Autodesk Inventor part; units mm, degrees
ref_plane "YZ Plane" through (0, 0, 0) normal (1, 0, 0) x (0, 1, 0)
ref_plane "XZ Plane" through (0, 0, 0) normal (0, 1, 0) x (-1, 0, 0)
ref_plane "XY Plane" through (0, 0, 0) normal (0, 0, 1) x (1, 0, 0)
sketch "Sketch1" plane through (0, 0, 0) normal (0, 0, 1) x (1, 0, 0)
  line L0 (-41.148, 14.2875) -> (41.148, 14.2875)
  line L1 (41.148, 14.2875) -> (41.148, -14.2875)
  line L2 (41.148, -14.2875) -> (-41.148, -14.2875)
  line L3 (-41.148, -14.2875) -> (-41.148, 14.2875)
  point P0 (0, 0)
  dimension "d0" = 82.296
  dimension "d1" = 41.148
  dimension "d2" = 14.2875
  dimension "d3" = 28.575
extrude "Extrusion1" add sketch "Sketch1" along normal mid plane 6.35
sketch "Sketch2" plane through (0, 0, 3.175) normal (0, 0, 1) x (1, 0, 0)
  circle A0 centre (-25.781, 0) radius 11.303
  circle A1 centre (0, 0) radius 11.303
  line L0 (41.148, -14.2875) -> (41.148, 14.2875)
  circle A2 centre (25.781, 0) radius 11.303
  line L1 (-41.148, 14.2875) -> (-41.148, -14.2875)
  line L2 (-41.148, 0) -> (41.148, 0) construction
  line L3 (41.148, 14.2875) -> (-41.148, 14.2875)
  point P0 (0, 0)
  dimension "d6" = 22.606
  dimension "d9" = 22.606
  dimension "d11" = 22.606
  dimension "d14" = 25.781
  dimension "d21" = 82.296
  dimension "d22" = 25.781
  dimension "d50" = 0
  dimension "d150" = 3.175
sketch "Sketch4" plane through (-41.148, -14.2875, -3.175) normal (-1, 0, 0) x (0, 0, 1)
  line L0 (0, 0) -> (0, 28.575)
  line L1 (6.35, 28.575) -> (6.35, 0)
  line L2 (0, 22.6695) -> (6.35, 22.6695)
  line L3 (6.35, 22.6695) -> (6.35, 5.9055)
  line L4 (6.35, 5.9055) -> (0, 5.9055)
  line L5 (0, 5.9055) -> (0, 22.6695)
  point P0 (3.175, 14.2875)
  dimension "d30" = 8.382
  dimension "d31" = 16.764
extrude "Extrusion3" cut sketch "Sketch4" against normal blind 0.635
mirror "Mirror1" about plane through (0, 0, 0) normal (1, 0, 0) of "Extrusion3"
sketch "Sketch5" plane through (0, 0, 3.175) normal (0, 0, 1) x (1, 0, 0)
  circle A0 centre (0, 9.7155) radius 3.175 construction
  line L0 (41.148, 14.2875) -> (-41.148, 14.2875)
  line L1 (-18.3944, 20.454) -> (40.513, 0) construction
  line L2 (40.513, 8.382) -> (40.513, -8.382)
  circle A1 centre (2.6968, 17.4822) radius 3.175 construction
  circle A2 centre (35.941, 1.5875) radius 3.175 construction
  circle A3 centre (-35.941, 26.5465) radius 3.175 construction
  line L3 (-40.513, 8.382) -> (-40.513, -8.382)
  circle A4 centre (36.576, 9.7155) radius 3.175
  circle A5 centre (-36.576, -9.7155) radius 3.175
  line L4 (41.148, 8.382) -> (41.148, 14.2875)
  line L5 (-41.148, -14.2875) -> (41.148, -14.2875)
  line L6 (-41.148, -14.2875) -> (-41.148, -8.382)
  point P0 (0, 0)
  dimension "d34" = 6.35
  dimension "d35" = 4.572
  dimension "d53" = 6.35
  dimension "d54" = 6.35
  dimension "d55" = 4.572
  dimension "d56" = 4.572
  dimension "d57" = 12.7
  dimension "d58" = 6.35
  dimension "d59" = 6.35
  dimension "d60" = 4.572
  dimension "d61" = 4.572
  dimension "d62" = 4.572
  dimension "d63" = 4.572
extrude "Extrusion4" cut sketch "Sketch5" against normal blind 1.27
sketch "Sketch7" plane through (-41.148, -14.2875, 3.175) normal (0, -1, 0) x (1, 0, 0)
  line L0 (27.178, -14.605) -> (55.118, -14.605)
  line L1 (55.118, -14.605) -> (55.118, 8.255)
  line L2 (55.118, 8.255) -> (27.178, 8.255)
  line L3 (27.178, 8.255) -> (27.178, -14.605)
  point P0 (41.148, -3.175)
  dimension "d39" = 27.94
  dimension "d40" = 22.86
  dimension "d41" = 11.43
  dimension "d42" = 13.97
extrude "Extrusion5" [suppressed]
sketch "Sketch8" plane through (0, 0, -3.175) normal (0, 0, -1) x (-1, 0, 0)
  line L0 (-41.148, 14.2875) -> (41.148, 14.2875)
  line L1 (15.6718, 14.2875) -> (-15.6718, 14.2875)
  line L2 (-15.6718, 14.2875) -> (-15.6718, 52.3875)
  line L3 (-15.6718, 52.3875) -> (15.6718, 52.3875)
  line L4 (15.6718, 52.3875) -> (15.6718, 14.2875)
  point P0 (0, 0)
  dimension "d45" = 31.3436
  dimension "d46" = 38.1
  dimension "d47" = 15.6718
extrude "Extrusion6" add sketch "Sketch8" against normal up to surface (6.35 mm away)
extrude "Extrusion7" cut sketch "Sketch2" against normal blind 25.4
sketch "Sketch9" plane through (-15.6718, 52.3875, -3.175) normal (0, 1, 0) x (1, 0, 0)
  line L0 (-25.4762, -6.35) -> (56.8198, -6.35)
  line L1 (3.1718, -6.35) -> (28.1718, -6.35)
  line L2 (28.1718, -6.35) -> (28.1718, -3.175)
  line L3 (28.1718, -3.175) -> (3.1718, -3.175)
  line L4 (3.1718, -3.175) -> (3.1718, -6.35)
  point P0 (15.6718, -3.175)
  dimension "d64" = 3.175
  dimension "d65" = 25
  dimension "d66" = 12.5
extrude "Extrusion8" [suppressed]
sketch "Sketch13" plane through (0, 0, 3.175) normal (0, 0, 1) x (1, 0, 0)
  line L0 (-41.148, -8.382) -> (-41.148, -14.2875)
  line L1 (-41.148, -14.2875) -> (41.148, -14.2875)
  line L2 (41.148, -14.2875) -> (41.148, -8.382)
  line L3 (41.148, -8.382) -> (40.513, -8.382)
  line L4 (-40.513, -8.382) -> (-41.148, -8.382)
  line L5 (-40.513, -8.382) -> (-40.513, 0)
  line L6 (-40.513, 8.382) -> (-40.513, -8.382)
  line L7 (-40.513, 0) -> (40.513, 0)
  line L8 (40.513, 8.382) -> (40.513, -8.382)
  line L9 (40.513, 0) -> (40.513, -8.382)
  point P0 (0, 0)
extrude "Extrusion11" cut sketch "Sketch13" against normal through all
sketch "Sketch14" plane through (37.084, 0, 3.175) normal (0, -1, 0) x (1, 0, 0)
  line L0 (3.429, -6.35) -> (0, -6.35)
  line L1 (3.429, 0) -> (3.429, -6.35)
  line L2 (0, 0) -> (3.429, 0)
  line L3 (0, -6.35) -> (0, 0)
  line L4 (-3.683, -1.27) -> (2.667, -1.27)
  circle A0 centre (1.7145, -3.81) radius 1.5494
  point P0 (-37.084, -3.175)
  dimension "d84" = 3.0988
  dimension "d85" = 6.35
  dimension "d86" = 5.08
  dimension "d87" = 3.429
  dimension "d88" = 1.7145
  dimension "d89" = 2.54
extrude "Extrusion12" cut sketch "Sketch14" against normal through all contours A0
mirror "Mirror3" about plane through (0, 0, 0) normal (1, 0, 0) of "Extrusion12"
thread "Thread3"
thread "Thread4"
sketch "Sketch15" plane through (-15.6718, 52.3875, -3.175) normal (0, 1, 0) x (1, 0, 0)
  line L0 (0, -6.35) -> (0, 0)
  line L1 (0, 0) -> (3.175, 0)
  line L2 (3.175, 0) -> (3.175, 5.08)
  line L3 (3.175, 5.08) -> (0, 5.08)
  line L4 (0, 5.08) -> (0, 0)
  line L5 (31.3436, 0) -> (0, 0) construction
  line L6 (11.5062, 0) -> (19.8374, 0)
  line L7 (31.3436, 0) -> (28.1686, 0)
  line L8 (28.1686, 0) -> (28.1686, 5.08)
  line L9 (28.1686, 5.08) -> (31.3436, 5.08)
  line L10 (31.3436, 5.08) -> (31.3436, 0)
  line L11 (31.3436, 0) -> (31.3436, -6.35)
  line L12 (4.3688, 0) -> (26.9748, 0)
  line L13 (19.8374, 0) -> (28.1686, 0)
  point P0 (15.6718, -3.175)
  point P1 (19.8374, 5.08)
  point P2 (3.175, 0.8467)
  dimension "d96" = 5.08
  dimension "d102" = 31.3436
  dimension "d105" = 3.175
  dimension "d106" = 3.175
  dimension "d120" = 5.08
sketch "Sketch16" plane through (-15.6718, 52.3875, 3.175) normal (0, 1, 0) x (1, 0, 0)
  line L0 (31.3436, 6.35) -> (0, 6.35)
  arc A0 (8.3312, 6.35) -> (11.5062, 6.35) centre (9.9187, 6.35) ccw
  line L1 (11.5062, 10.5833) -> (11.5062, 6.35)
  line L2 (8.3312, 6.35) -> (8.3312, 10.5833)
  line L3 (4.3688, 6.35) -> (26.9748, 6.35)
  arc A1 (19.8374, 6.35) -> (23.0124, 6.35) centre (21.4249, 6.35) ccw
  line L4 (23.0124, 10.5833) -> (23.0124, 6.35)
  line L5 (19.8374, 6.35) -> (19.8374, 10.5833)
  point P0 (15.6718, 3.175)
extrude "Extrusion15" [suppressed]
fillet "Fillet3" [suppressed]
fillet "Fillet4" [suppressed]
fillet "Fillet5" radius 3.175 2 edges at (15.6718, 14.2875, 0) (-15.6718, 14.2875, 0)
extrude "Extrusion16" add sketch "Sketch15" against normal blind 40.64
sketch "Sketch17" plane through (-15.6718, 52.3875, 3.175) normal (0, 1, 0) x (1, 0, 0)
  line L0 (28.1686, 6.35) -> (28.1686, 11.43)
  line L1 (3.175, 11.43) -> (3.175, 6.35)
  line L2 (28.1686, 11.43) -> (3.175, 11.43)
  line L3 (3.175, 11.43) -> (3.175, 6.35)
  line L4 (3.175, 6.35) -> (28.1686, 6.35)
  line L5 (28.1686, 6.35) -> (28.1686, 11.43)
  point P0 (15.6718, 3.175)
extrude "Extrusion17" add sketch "Sketch17" against normal blind 3.175
fillet "Fillet6" radius 3.175 2 edges at (-12.4968, 49.2125, -5.715) (12.4968, 49.2125, -5.715)
sketch "Sketch18" plane through (-15.6718, 52.3875, 3.175) normal (0, 1, 0) x (1, 0, 0)
  circle A0 centre (9.2964, 8.89) radius 1.6764
  circle A1 centre (22.0472, 8.89) radius 1.6764
  line L0 (31.3436, 11.43) -> (0, 11.43)
  line L1 (6.35, 6.35) -> (24.9936, 6.35)
  line L2 (6.35, 11.43) -> (6.35, 6.35)
  line L3 (24.9936, 6.35) -> (24.9936, 11.43)
  line L4 (7.62, 8.89) -> (23.7236, 8.89) construction
  point P0 (15.6718, 3.175)
  point P1 (23.7236, 8.89)
  dimension "d126" = 3.3528
  dimension "d127" = 3.3528
  dimension "d128" = 5.08
  dimension "d129" = 2.54
  dimension "d130" = 2.54
  dimension "d132" = 1.27
  dimension "d134" = 1.27
extrude "Extrusion18" cut sketch "Sketch18" against normal through all contours A0 | A1
sketch "Sketch19" plane through (-15.6718, 52.3875, 3.175) normal (0, 1, 0) x (1, 0, 0)
  line L0 (6.35, 6.35) -> (24.9936, 6.35)
  line L1 (0, 0) -> (31.3436, 0)
  circle A0 centre (15.6718, 3.175) radius 1.6764
  dimension "d137" = 3.3528
extrude "Extrusion19" cut sketch "Sketch19" against normal blind 12.7
thread "Thread5"
sketch "Sketch20" plane through (-15.6718, 52.3875, 3.175) normal (0, 1, 0) x (1, 0, 0)
  circle A0 centre (9.2964, 8.89) radius 1.6764
  circle A1 centre (15.6718, 3.175) radius 1.6764
  circle A2 centre (9.2964, 8.89) radius 1.6764
  circle A3 centre (22.0472, 8.89) radius 1.6764
  line L0 (0, 0) -> (31.3436, 0)
  line L1 (31.3436, 11.43) -> (31.3436, 0)
  line L2 (31.3436, 11.43) -> (0, 11.43)
  line L3 (0, 11.43) -> (0, 0)
  dimension "d142" = 2.54
  dimension "d143" = 9.2964
  dimension "d144" = 8.255
equation "\"d9\" = d7"
equation "\"d11\" = d9"
equation "\"d22\" = d14"
equation "\"d88\" = 0.5 * d87"
equation "\"d89\" = 0.5 * d86"
equation "\"d106\" = d105"
equation "\"d120\" = d96"
equation "\"d127\" = d126"
equation "\"d130\" = 0.5 * d128"
equation "\"d134\" = d132"
equation "\"d7\" = d6"
properties part number "Tube Holder with camera attachment" material "Aluminum 6061-AHC"
Design review of the part built by this model. Coordinates are the model's own, in mm. A direction names the side the tool comes from. Round coordinates to 2 decimals unless told otherwise and drop trailing zeros. Order: outer loops, then holes, each group sorted by start corner. A loop starts at its lowest first (then second) coordinate and runs counter-clockwise, first axis right, second up. Notation, with made-up numbers: M 56.5,-9 L 91.5,-9 A25 ccw 91.5,18 Z; hole C -39,31.5 d10. An arc over 180 degrees is marked long. Answer as CSV lines item,"result". Start each with the question number.
1) Add section B-B (y = 42). Give the boundary of the cut face in (x, z) (3 decimals), then the cut area to 3 significant figures.
2) For pin 1 Ø4 at (x, z) = (38.8, -0.64) entering from +Y; pin 2 Ø2 at (x, z) = (-22, 0) entering from -Y; pin 3 Ø5.5 at (y, z) = (35, -5.5) entering from +X, all flat-tipped, find the tip position at first contact; note any pin that passes through.
3) Tool access review of faces 1 (the face through (-40.513, 4, 0)), 2 (the face through (40.513, 4, 0)), 3 (the face through (30, 14.288, 0)), 4 (the face through (12.497, 29, -6)): name each direction out of +Z, -Z, +X, -X, +Y, -Y from which nothing blocks a thin tool from reaching the whole face with its end or side.
4) The part is to be moulded in two halves that separate along Z. For faces 5 (the face through (0, 28, 3.175)), 6 (the face through (-30, 14.288, 0)), 7 (the face through (0, 39.688, 0)), say which applies: +Z half, -Z half, draft (parallel to the pull), parting line (faces both ways), or undercut.
5) Add section C-C (y = 28.5). Give the boundary of the cut face in (x, z) (3 decimals), then the cut area to 3 significant figures.
6) Add section A-A (y = 4.5). Give the boundary of the cut face in (x, z) (1 decimal).
7) Add section D-D (x = -3.5). Give the boundary of the cut face in (y, z) (1 decimal).
8) Wall thickness on line 1 along X through (y, z) = (30.5, -6.75); line 2 along Z through (x, y) = (0, 44) (3 decimals); line 3 along Z through (x, y) = (-4.5, 14) (3 decimals): over which ranges is each line inside the solid? List them lowest first. Write a range as [from, to].
Resolved:
1,outline,"M -15.672,-8.255 L -12.497,-8.255 L -12.497,-3.175 L 12.497,-3.175 L 12.497,-8.255 L 15.672,-8.255 L 15.672,3.175 L -15.672,3.175 Z; hole C 0,0 d3.353"
1,area,"222 mm^2"
2,pin 1,"y = 14.29"
2,pin 2,"y = 10.24"
2,pin 3,"x = 15.67"
3,face 1,"+Z, -Z, -X, -Y"
3,face 2,"+Z, -Z, +X, -Y"
3,face 3,"+Z, -Z, +X, +Y"
3,face 4,"-Z, -Y"
4,face 5,"+Z half"
4,face 6,"draft"
4,face 7,"undercut"
5,outline,"M -15.672,-8.255 L -12.497,-8.255 L -12.497,-3.175 L 12.497,-3.175 L 12.497,-8.255 L 15.672,-8.255 L 15.672,3.175 L -15.672,3.175 Z"
5,area,"231 mm^2"
6,outline,"M -40.5,-3.2 L -36.1,-3.2 L -36.1,3.2 L -40.5,3.2 Z; M -15.4,-3.2 L -10.4,-3.2 L -10.4,3.2 L -15.4,3.2 Z; M 10.4,-3.2 L 15.4,-3.2 L 15.4,3.2 L 10.4,3.2 Z; M 36.1,-3.2 L 40.5,-3.2 L 40.5,3.2 L 36.1,3.2 Z; hole C -38.8,-0.6 d3.1; hole C 38.8,-0.6 d3.1"
7,outline,"M 10.7,-3.2 L 49.2,-3.2 L 49.2,-8.3 L 52.4,-8.3 L 52.4,3.2 L 10.7,3.2 Z"
8,line 1,"[-15.67, -12.5], [12.5, 15.67]"
8,line 2,"[-3.175, -1.676], [1.676, 3.175]"
8,line 3,"[-3.175, 3.175]"
